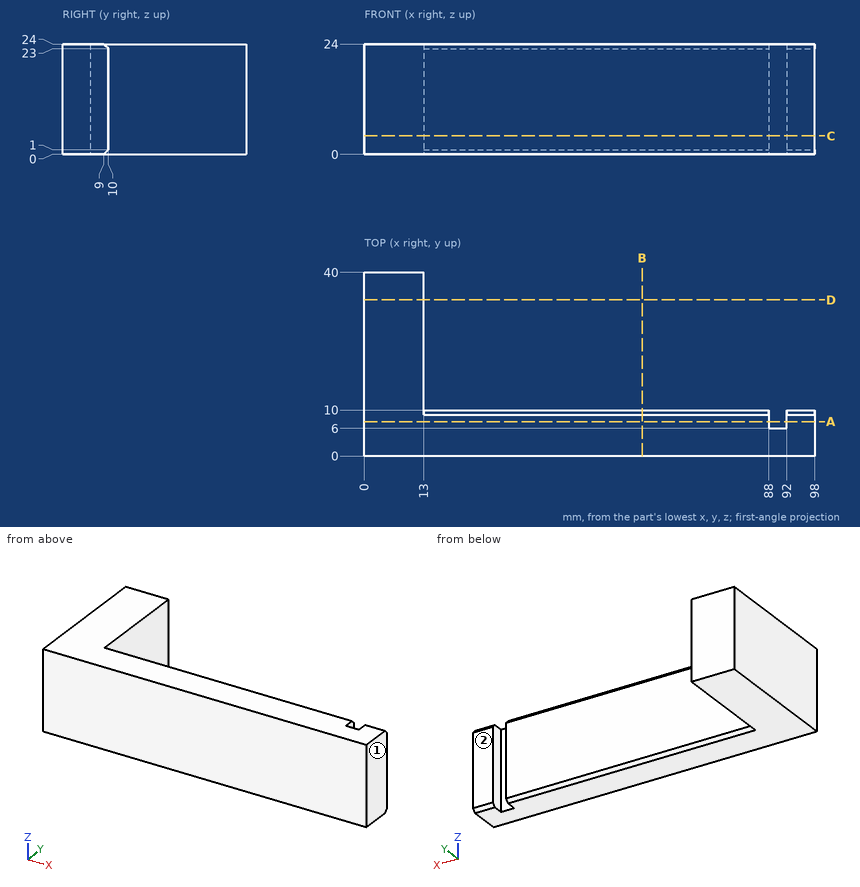
Design review of the part shown in the three views and the two pictorial views. Dimensions are in mm from the part's minimum x, y and z. A direction names the side the tool comes from. Give positions to 0.01 mm unless a question says otherwise; leave off trailing zeros. Write each loop counter-clockwise with the first axis right and the second up, starting at its lowest first coordinate (ties: lowest second). Pieces come first, ordered by that corner, then holes. Notation, with made-up numbers: M 59,3.25 L 117,3.25 A32 cw 117,39.25 Z; hole C 36.25,20 d9. An arc over 180 degrees is marked long. Return JSON: item names as keys, results as strings. Group by question number.
Item 1: Take a section at D-D (y = 34). Give the boundary of the cut face in (x, z).
Item 2: Tool access review of the marked faces 1 and 2: name each direction out of +Z, -Z, +X, -X, +Y, -Y from which nothing blocks a thin tool from reaching the whole face with its end or side.
Item 3: Take a section at B-B (x = 60.5). Give the boundary of the cut face in (y, z).
Item 4: Take a section at A-A (y = 7.5). Give the boundary of the cut face in (x, z).
Item 5: Take a section at C-C (z = 4). Give the boundary of the cut face in (x, y), plus the area to 3 significant figures.
Item 6: Wall thickness on line 1 along Y through (x, z) = (62, 3.75); line 2 along X through (y, z) = (7.5, 7.75); line 3 along X through (y, z) = (14, 7.5): over which ranges is each line inside the solid? List them lowest first.
Item 7: Clearance check with flat-ended pins moving along their axes: pin 1 Ø4 at (x, z) = (68, 7) entering from +Y; pin 2 Ø7 at (y, z) = (24, 8.5) entering from +X. State where each tip first meets the part, or that it passes through.
Return value:
{
 "1": {"outline": "M 0,0 L 13,0 L 13,24 L 0,24 Z"},
 "2": {"face 1": "+Z, -Z, +X, +Y, -Y", "face 2": "+Z, -Z, +X, +Y"},
 "3": {"outline": "M 0,0 L 9,0 L 10,1 L 10,23 L 9,24 L 0,24 Z"},
 "4": {"outline": "M 0,0 L 88,0 L 88,24 L 0,24 Z; M 92,0 L 98,0 L 98,24 L 92,24 Z"},
 "5": {"outline": "M 0,0 L 98,0 L 98,10 L 92,10 L 92,6 L 88,6 L 88,10 L 13,10 L 13,40 L 0,40 Z", "area": "1,350 mm2"},
 "6": {"line 1": "y = 0 to 10", "line 2": "x = 0 to 88, 92 to 98", "line 3": "x = 0 to 13"},
 "7": {"pin 1": "stops at y = 10", "pin 2": "stops at x = 13"}
}
